Verification items for the finished model (mm, model axes). A direction names the side the tool comes from. Give positions to 0.01 mm unless a question says otherwise; leave off trailing zeros. Write each loop counter-clockwise with the first axis right and the second up, starting at its lowest first coordinate (ties: lowest second). Pieces come first, ordered by that corner, then holes. Notation, with made-up numbers: M 8.5,7 L 66.5,7 A24 ccw 66.5,36 Z; hole C 12.25,-3.75 d2. An arc over 180 degrees is marked long. Answer as a JSON object with one key per item and string values.
```python
from build123d import *

# Parameters (mm, degrees)
SKETCH1_R               = 50
BOSS_EXTRUDE1_DEPTH     = 1.5
SKETCH2_R               = 50
SKETCH2_W               = 57.15
SKETCH2_H               = 28.15
BOSS_EXTRUDE2_DEPTH     = 1.415
BOSS_EXTRUDE3_START     = 5
BOSS_EXTRUDE3_DEPTH     = 5
CUT_EXTRUDE1_DEPTH      = 71.887234394
CUT_EXTRUDE1_DEPTH_BACK = 71.887234394
SKETCH6_W               = 1.8
SKETCH6_H               = 4.5
BOSS_EXTRUDE4_DEPTH     = 3.5
SKETCH7_W               = 1.8
SKETCH7_H               = 4.5
BOSS_EXTRUDE5_DEPTH     = 3.5
SKETCH8_W               = 30.276808401
SKETCH8_H               = 9.415
SKETCH8_W_2             = 41.626808401
BOSS_EXTRUDE6_DEPTH     = 2
SKETCH9_W               = 28.15
SKETCH9_H               = 1.915
CUT_EXTRUDE3_DEPTH      = 0.5
FILLET1_START           = -2
FILLET1_DEPTH           = 11
FILLET1_START_2         = -1.5
FILLET1_2_DEPTH         = 9.415


with BuildPart() as part:
    # Sketch1 → Boss-Extrude1 (new, symmetric)
    with BuildSketch(Plane(origin=(0, 0, 0), x_dir=(1, 0, 0), z_dir=(0, 1, 0))):
        with Locations(Location((0, 0, 0), (0, 0, 270))):
            Circle(SKETCH1_R)
    extrude(amount=BOSS_EXTRUDE1_DEPTH, both=True)

    # Sketch2 → Boss-Extrude2 (add, symmetric)
    with BuildSketch(Plane(origin=(0, 1.5, 0), x_dir=(1, 0, 0), z_dir=(0, 1, 0))):
        with Locations(Location((0, 0, 0), (0, 0, 270))):
            Circle(SKETCH2_R)
        with Locations((-10.265, 5.675)):
            Rectangle(SKETCH2_W, SKETCH2_H, mode=Mode.SUBTRACT)
    extrude(amount=BOSS_EXTRUDE2_DEPTH, both=True)

    # Sketch3 → Boss-Extrude3 (add)
    with BuildSketch(Plane(origin=(0, 2.915, 0), x_dir=(1, 0, 0), z_dir=(0, 1, 0)).offset(BOSS_EXTRUDE3_START)):
        with BuildLine():
            Line((16.51, 45.284212481), (16.51, 19.75))
            Line((16.51, 19.75), (18.31, 19.75))
            Line((18.31, 19.75), (18.31, 46.526808401))
            ThreePointArc((18.31, 46.526808401), (-50, 0), (18.31, -46.526808401))
            Line((18.31, -46.526808401), (18.31, -8.4))
            Line((18.31, -8.4), (16.51, -8.4))
            Line((16.51, -8.4), (16.51, -45.284212481))
            ThreePointArc((16.51, -45.284212481), (-48.2, 0), (16.51, 45.284212481))
        make_face()
    extrude(amount=-BOSS_EXTRUDE3_DEPTH)

    # Sketch4 → Cut-Extrude1 (cut, two sides: drawn at the far end of the back side and taken through both)
    with BuildSketch(Plane(origin=(0, 2.915, 0), x_dir=(1, 0, 0), z_dir=(0, 1, 0)).offset(-CUT_EXTRUDE1_DEPTH_BACK)):
        with BuildLine():
            Line((18.31, -46.526808401), (18.31, 46.526808401))
            ThreePointArc((18.31, 46.526808401), (50, 0), (18.31, -46.526808401))
        make_face()
    extrude(amount=CUT_EXTRUDE1_DEPTH + CUT_EXTRUDE1_DEPTH_BACK, mode=Mode.SUBTRACT)

    # Sketch6 → Boss-Extrude4 (add)
    with BuildSketch(Plane.XY.offset(-19.75)):
        with Locations((17.41, 5.665)):
            Rectangle(SKETCH6_W, SKETCH6_H)
    extrude(amount=BOSS_EXTRUDE4_DEPTH)

    # Sketch7 → Boss-Extrude5 (add)
    with BuildSketch(Plane(origin=(0, 0, 8.4), x_dir=(-1, 0, 0), z_dir=(0, 0, -1))):
        with Locations((-17.41, 5.665)):
            Rectangle(SKETCH7_W, SKETCH7_H)
    extrude(amount=BOSS_EXTRUDE5_DEPTH)

    # Sketch8 → Boss-Extrude6 (add)
    with BuildSketch(Plane(origin=(18.31, 0, 0), x_dir=(0, 0, -1), z_dir=(1, 0, 0))):
        with Locations((31.388404201, 3.2075)):
            Rectangle(SKETCH8_W, SKETCH8_H)
        with Locations((-25.713404201, 3.2075)):
            Rectangle(SKETCH8_W_2, SKETCH8_H)
    extrude(amount=BOSS_EXTRUDE6_DEPTH)

    # Sketch9 → Cut-Extrude3 (cut)
    with BuildSketch(Plane.ZY.offset(-18.31)):
        with Locations((-5.675, 2.4575)):
            Rectangle(SKETCH9_W, SKETCH9_H)
    extrude(amount=-CUT_EXTRUDE3_DEPTH, mode=Mode.SUBTRACT)

    # Fillet1: read off the stored shape, not the designer's step
    # Fillet1 outline → Fillet1 (cut)
    with BuildSketch(Plane(origin=(0, 0, 0), x_dir=(1, 0, 0), z_dir=(0, 1, 0)).offset(FILLET1_START)):
        with BuildLine():
            Line((20.31, -4.9), (18.81, -4.9))
            ThreePointArc((18.81, -4.9), (19.870660172, -5.339339828), (20.31, -6.4))
            Line((20.31, -6.4), (20.31, -4.9))
        make_face()
        with BuildLine():
            Line((20.31, 16.25), (20.31, 17.75))
            ThreePointArc((20.31, 17.75), (19.870660172, 16.689339828), (18.81, 16.25))
            Line((18.81, 16.25), (20.31, 16.25))
        make_face()
        with BuildLine():
            Line((20.31, 46.526808401), (18.81, 46.526808401))
            ThreePointArc((18.81, 46.526808401), (19.870660172, 46.087468573), (20.31, 45.026808401))
            Line((20.31, 45.026808401), (20.31, 46.526808401))
        make_face()
        with BuildLine():
            Line((20.31, -46.526808401), (20.31, -45.026808401))
            ThreePointArc((20.31, -45.026808401), (19.870660172, -46.087468573), (18.81, -46.526808401))
            Line((18.81, -46.526808401), (20.31, -46.526808401))
        make_face()
    extrude(amount=FILLET1_DEPTH, mode=Mode.SUBTRACT)

    # Fillet1 2 outline → Fillet1 2 (add)
    with BuildSketch(Plane(origin=(0, 0, 0), x_dir=(1, 0, 0), z_dir=(0, 1, 0)).offset(FILLET1_START_2)):
        with BuildLine():
            ThreePointArc((18.592355278, 46.526808401), (18.316908931, 46.552315502), (18.050830367, 46.627969322))
            ThreePointArc((18.050830367, 46.627969322), (18.180485544, 46.577569122), (18.31, 46.526808401))
            Line((18.31, 46.526808401), (18.592355278, 46.526808401))
        make_face()
        with BuildLine():
            ThreePointArc((18.050830367, -46.627969322), (18.316908931, -46.552315502), (18.592355278, -46.526808401))
            Line((18.592355278, -46.526808401), (18.31, -46.526808401))
            ThreePointArc((18.31, -46.526808401), (18.180485544, -46.577569122), (18.050830367, -46.627969322))
        make_face()
    extrude(amount=FILLET1_2_DEPTH)


solid = part.part
```
1) Thickness scan on L1, parallel to Z at x = 0, y = 5.2; L2, parallel to Y at x = -8, z = 3.5; L3, parallel to Y at x = -34.5, z = 9 (3 decimals). Record the ranges inside material, lowest first.
Completed:
{"L1": "z = -50 to -48.2, 48.2 to 50", "L2": "y = -1.5 to 1.5", "L3": "y = -1.5 to 2.915"}
2) Section check D-D on x = -26.5. Record the boundary of the cut face in (y, z) (3 decimals), and give its area (3 significant figures).
Completed:
{"outline": "M -1.5,-42.4 L 7.915,-42.4 L 7.915,-40.262 L 2.915,-40.262 L 2.915,-19.75 L 1.5,-19.75 L 1.5,8.4 L 2.915,8.4 L 2.915,40.262 L 7.915,40.262 L 7.915,42.4 L -1.5,42.4 Z", "area": "356 mm2"}
3) Section check C-C on y = 6.5. Record the boundary of the cut face in (x, z), and give its area (3 significant figures).
Completed:
{"outline": "M 16.51,-45.28 A48.2 cw long 16.51,45.28 L 16.51,4.9 L 18.81,4.9 A1.5 ccw 20.31,6.4 L 20.31,45.03 A1.5 ccw 18.81,46.53 L 18.59,46.53 A1.5 cw 18.05,46.63 A50 ccw long 18.05,-46.63 A1.5 cw 18.59,-46.53 L 18.81,-46.53 A1.5 ccw 20.31,-45.03 L 20.31,-17.75 A1.5 ccw 18.81,-16.25 L 16.51,-16.25 Z", "area": "611 mm2"}
4) Section check A-A on x = 0. Record the boundary of the cut face in (y, z) (3 decimals), and give its area (3 significant figures).
Completed:
{"outline": "M -1.5,-50 L 7.915,-50 L 7.915,-48.2 L 2.915,-48.2 L 2.915,-19.75 L 1.5,-19.75 L 1.5,8.4 L 2.915,8.4 L 2.915,48.2 L 7.915,48.2 L 7.915,50 L -1.5,50 Z", "area": "420 mm2"}
5) Release check for a two-part mould opening along Z. For faces 6 (the face through (18, 3.415, 7)), 7 (the face through (19, 7.915, 7)) record: pulls with the +Z half, pulls with the -Z half, needs draft (parallel to the pull), parting line crosses it, or undercut.
Completed:
{"face 6": "undercut", "face 7": "needs draft"}
6) Access from +Z, -Z, +X, -X, +Y, -Y to the whole of each face (thin tool, end or side, straight path). Record for faces 1 (the face through (16.51, 5, -31)), 2 (the face through (18, 3.415, -18)), 3 (the face through (20.31, 3, -31)), 4 (the face through (18.31, 0, -6)), 5 (the face through (18, 6, 4.9)).
Completed:
{"face 1": "+Y", "face 2": "none", "face 3": "+Z, -Z, +X, +Y, -Y", "face 4": "+X, +Y, -Y", "face 5": "+X, +Y"}
7) Section check B-B on z = 0. Record the boundary of the cut face in (x, y) (3 decimals), and give its area (3 significant figures).
Completed:
{"outline": "M -50,-1.5 L 18.31,-1.5 L 18.31,1.5 L -38.84,1.5 L -38.84,2.915 L -48.2,2.915 L -48.2,7.915 L -50,7.915 Z", "area": "230 mm2"}
8) Go/stop test with flat-tipped pins: pin 1 (0.6 mm diameter, centred on x = 3, y = 3, fed in from -Z); pin 2 (0.7 mm diameter, centred on x = 18, y = 5, fed in from -Z); pin 3 (1 mm diameter, centred on x = -10, y = 6.5, fed in from +Z). Record where each tip stops, or that it passes through.
Completed:
{"pin 1": "stops at z = -49.93", "pin 2": "stops at z = -46.78", "pin 3": "stops at z = 49.09"}
